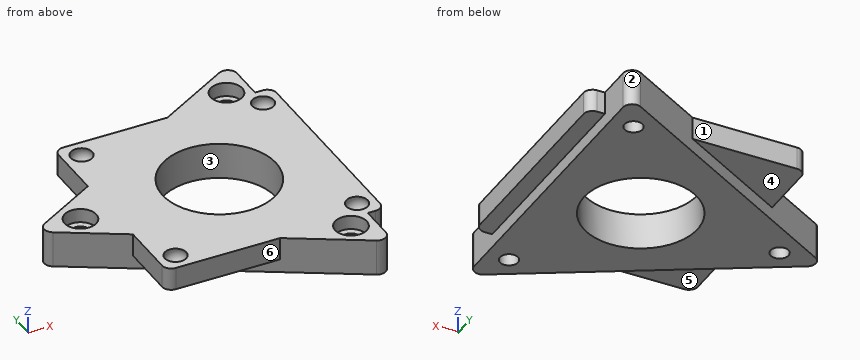
Autodesk Inventor part; units mm, degrees
ref_plane "YZ Plane" through (0, 0, 0) normal (1, 0, 0) x (0, 1, 0)
ref_plane "XZ Plane" through (0, 0, 0) normal (0, 1, 0) x (-1, 0, 0)
ref_plane "XY Plane" through (0, 0, 0) normal (0, 0, 1) x (1, 0, 0)
sketch "Sketch1" plane through (0, 0, 0) normal (0, 0, 1) x (1, 0, 0)
  line L0 (15.2998, 26.5) -> (15.2998, -26.5) construction
  line L1 (15.2998, -26.5) -> (-30.5996, 0) construction
  line L2 (-30.5996, 0) -> (15.2998, 26.5) construction
  line L3 (0, 48.0119) -> (0, -48.0119)
  circle A0 centre (0, 0) radius 12.5
  line L4 (24.9, -24.45) -> (-24.9, -24.45) construction
  line L5 (-24.9, -24.45) -> (-24.9, 24.45) construction
  line L6 (-24.9, 24.45) -> (24.9, 24.45) construction
  line L7 (24.9, 24.45) -> (24.9, -24.45) construction
  line L8 (24.9, -24.45) -> (-24.9, 24.45) construction
  line L9 (-24.9, -24.45) -> (24.9, 24.45) construction
  line L10 (20, -20) -> (-20, -20) construction
  line L11 (-20, -20) -> (-20, 20) construction
  line L12 (-20, 20) -> (20, 20) construction
  line L13 (20, 20) -> (20, -20) construction
  line L14 (20, -20) -> (-20, 20) construction
  line L15 (-20, -20) -> (20, 20) construction
  line L16 (-37.5996, -1.7321) -> (17.2998, -33.4282)
  line L17 (20.2998, -31.6962) -> (20.2998, 31.6962)
  line L18 (17.2998, 33.4282) -> (-37.5996, 1.7321)
  arc A1 (-37.5996, 1.7321) -> (-37.5996, -1.7321) centre (-36.5996, 0) ccw
  arc A2 (20.2998, 31.6962) -> (17.2998, 33.4282) centre (18.2998, 31.6962) ccw
  arc A3 (17.2998, -33.4282) -> (20.2998, -31.6962) centre (18.2998, -31.6962) ccw
  circle A4 centre (15.2998, 26.5) radius 2
  circle A5 centre (-30.5996, 0) radius 2
  circle A6 centre (15.2998, -26.5) radius 2
  dimension "d1" = 53
  dimension "d2" = 25
  dimension "d3" = 49.8
  dimension "d4" = 48.9
  dimension "d5" = 40
  dimension "d6" = 40
  dimension "d7" = 5
  dimension "d8" = 2
  dimension "d9" = 4
  dimension "d10" = 4
  dimension "d11" = 4
extrude "Extrusion1" add sketch "Sketch1" along normal blind 3 contours L18 A2 L17 A3 L16 L3 A0 | L3 A0 L16 A1 L18
sketch "Sketch3" plane through (0, 0, 3) normal (0, 0, 1) x (1, 0, 0)
  circle A0 centre (0, 0) radius 12.5
  circle A1 centre (15.2998, -26.5) radius 2
  circle A2 centre (-30.5996, 0) radius 2
  circle A3 centre (15.2998, 26.5) radius 2
  line L0 (-37.5996, -1.7321) -> (17.2998, -33.4282)
  arc A4 (17.2998, -33.4282) -> (20.2998, -31.6962) centre (18.2998, -31.6962) ccw
  line L1 (20.2998, -31.6962) -> (20.2998, 31.6962)
  arc A5 (20.2998, 31.6962) -> (17.2998, 33.4282) centre (18.2998, 31.6962) ccw
  line L2 (17.2998, 33.4282) -> (-37.5996, 1.7321)
  arc A6 (-37.5996, 1.7321) -> (-37.5996, -1.7321) centre (-36.5996, 0) ccw
  line L3 (22, -24) -> (-22, -24)
  line L4 (-24, -22) -> (-24, 22)
  line L5 (-22, 24) -> (22, 24)
  line L6 (24, 22) -> (24, -22)
  line L7 (24, -24) -> (-24, 24) construction
  line L8 (-24, -24) -> (24, 24) construction
  arc A7 (-22, 24) -> (-24, 22) centre (-22, 22) ccw
  arc A8 (-24, -22) -> (-22, -24) centre (-22, -22) ccw
  arc A9 (22, -24) -> (24, -22) centre (22, -22) ccw
  arc A10 (24, 22) -> (22, 24) centre (22, 22) ccw
  line L9 (17.2998, 33.4282) -> (-37.5996, 1.7321)
  line L10 (-37.5996, -1.7321) -> (17.2998, -33.4282)
  line L11 (20.2998, -31.6962) -> (20.2998, 31.6962)
  point P0 (20.2998, 24)
  point P1 (-24, 9.5838)
  point P2 (-24, -9.5838)
  point P3 (0.9697, -24)
  point P4 (20.2998, -24)
  dimension "d14" = 48
  dimension "d15" = 48
  dimension "d16" = 2
extrude "Extrusion2" add sketch "Sketch3" along normal blind 5 contours A0 | A1 | A3 | A6 L2 L4 L0 | L4 L2 L5 L1 L3 L0 | L0 L3 A8 L4 | L3 L1 A4 L0 | L4 A7 L5 L2 | L1 L5 A10 L6 A9 L3 | L2 A5 L1 L5
sketch "Sketch4" plane through (0, 0, 8) normal (0, 0, 1) x (1, 0, 0)
  circle A0 centre (0, 0) radius 12.5
  line L0 (20, -20) -> (-20, -20) construction
  line L1 (-20, -20) -> (-20, 20) construction
  line L2 (-20, 20) -> (20, 20) construction
  line L3 (20, 20) -> (20, -20) construction
  line L4 (20, -20) -> (-20, 20) construction
  line L5 (-20, -20) -> (20, 20) construction
  circle A1 centre (15.2998, 26.5) radius 2
  circle A2 centre (15.2998, -26.5) radius 2
  dimension "d19" = 40
  dimension "d20" = 40
extrude "Extrusion3" cut sketch "Sketch4" against normal through all
ref_plane "Work Plane1" through (-22, 0, 3) normal (0, 1, 0) x (1, 0, 0)
ref_plane "Work Plane2" through (0, -22, 3) normal (-1, 0, 0) x (0, 0, 1)
ref_plane "Work Plane3" through (-22, -20, 3) normal (0, 1, 0) x (1, 0, 0)
sketch "Sketch5" plane through (-22, -20, 3) normal (0, 1, 0) x (1, 0, 0)
  line L0 (22.9697, 0) -> (22.9697, -5)
  line L1 (22.9697, 0) -> (0, 0)
  line L2 (0, 0) -> (0, -5)
  line L3 (22.9697, -5) -> (0, -5)
  circle A0 centre (2, -4.2) radius 2.5
  line L4 (22, -11.7547) -> (22, 5.4591)
  line L5 (-0.5, -4.2) -> (4.5, -4.2)
  line L6 (0, 0) -> (0, -5)
  point P0 (22, 3)
  dimension "d24" = 5
  dimension "d25" = 20
  dimension "d26" = 0.8
revolve "Revolution1" cut sketch "Sketch5" angle 360 about axis through (-22.5, -20, 7.2) along (1, 0, 0) contours A0 L5 L2 L3 | L3 L2 L5 A0
pattern_linear "Rectangular Pattern1" count 2 spacing 40 along (1, 0, 0) count 2 spacing 40 along (0, 1, 0) of "Revolution1"
sketch "Sketch6" plane through (0, 0, 8) normal (0, 0, 1) x (1, 0, 0)
  circle A0 centre (20, 20) radius 2.3685
  circle A1 centre (-20, 20) radius 2.3685
  circle A2 centre (20, -20) radius 2.3685
  circle A3 centre (-20, -20) radius 2.3685
  circle A4 centre (15.2998, -26.5) radius 2
  circle A5 centre (15.2998, 26.5) radius 2
  circle A6 centre (0, 0) radius 12.5
  circle A7 centre (-30.5996, 0) radius 2
  line L0 (0.9697, 24) -> (-22, 24)
  arc A8 (-22, 24) -> (-24, 22) centre (-22, 22) ccw
  line L1 (-24, 22) -> (-24, 9.5838)
  line L2 (-24, 9.5838) -> (-37.5996, 1.7321)
  arc A9 (-37.5996, 1.7321) -> (-37.5996, -1.7321) centre (-36.5996, 0) ccw
  line L3 (-37.5996, -1.7321) -> (-24, -9.5838)
  line L4 (-24, -9.5838) -> (-24, -22)
  arc A10 (-24, -22) -> (-22, -24) centre (-22, -22) ccw
  line L5 (-22, -24) -> (0.9697, -24)
  line L6 (0.9697, -24) -> (17.2998, -33.4282)
  arc A11 (17.2998, -33.4282) -> (20.2998, -31.6962) centre (18.2998, -31.6962) ccw
  line L7 (20.2998, -31.6962) -> (20.2998, -24)
  line L8 (20.2998, -24) -> (22, -24)
  arc A12 (22, -24) -> (24, -22) centre (22, -22) ccw
  line L9 (24, -22) -> (24, 22)
  arc A13 (24, 22) -> (22, 24) centre (22, 22) ccw
  line L10 (22, 24) -> (20.2998, 24)
  line L11 (20.2998, 24) -> (20.2998, 31.6962)
  arc A14 (20.2998, 31.6962) -> (17.2998, 33.4282) centre (18.2998, 31.6962) ccw
  line L12 (17.2998, 33.4282) -> (0.9697, 24)
hole "Hole1" at (15.2998, 26.5, 8) at (15.2998, -26.5, 8) at (-30.5996, 0, 8) direction (0, 0, -1) diameter 2.8 depth 30 tip angle 118 counterbore diameter 7 counterbore depth 3.1
properties part number "20_Cube_Insert_Openflexure_Deltastage_Adapter"
Source: CAD feature listing. Evaluate the final solid. Frame: model axes, mm. Face numbers are marked on the shaded views. A direction names the side the tool comes from. Coordinates: 2 decimals unless noted, no trailing zeros. Loops run counter-clockwise (first coordinate to the right, second up) from the corner with the lowest first, then second, coordinate; pieces in that order, holes last. Notation, with made-up numbers: M 15,6 L 64,6 A22 cw 64,24 Z; hole C -20,74 d11. An arc over 180 degrees is marked long. Put each result on its own line as item: value. Start each with the question number.
1) Reachability of the marked faces 4, 5 and 6 from +Z, -Z, +X, -X, +Y, -Y: full face, straight path, thin tool, end or side. Return the list, or none.
2) Cut plane D-D on y = 26.5. Return the cut outline in (x, z), then the cut area to 3 significant figures.
3) Cut plane B-B on x = 0. Return the cut outline in (y, z).
4) Ray query, L1, parallel to Y at x = -0.5, z = 3.75; L2, parallel to X at y = -21.5, z = 5.5; L3, parallel to Y at x = 18.5, z = 6. Return the intervals inside material, ascending. Write a range as from..to.
5) Cut plane A-A on y = 0. Return the cut outline in (x, z).
6) Contact query for flat-ended pins moving along their axis: pin 1 Ø2 at (x, z) = (-28, 7) entering from +Y; pin 2 Ø4 at (y, z) = (-14.5, 4.5) entering from -X; pin 3 Ø5.5 at (x, y) = (15.3, 26.5) entering from +Z. Output: stop coordinate, or through.
7) Cut plane C-C on z = 1.75. Return the cut outline in (x, y), then the cut area to 3 significant figures.
8) Pull-direction query (X, two-part tool) for the marked faces 1, 2 and 3; classes: pulls with the +X half, pulls with the -X half, needs draft (parallel to the pull), parting line crosses it, or undercut.
The answers:
1. face 4: -Z, -X, +Y
1. face 5: -Z, -X, -Y
1. face 6: +Z, -Z, -X, -Y
2. outline: M 5.3,0 L 13.3,0 L 13.3,4.9 L 11.8,4.9 L 11.8,8 L 5.3,8 Z; M 17.3,0 L 20.3,0 L 20.3,8 L 18.8,8 L 18.8,4.9 L 17.3,4.9 Z
2. area: 78.7 mm²
3. outline: M -24,3 L -23.44,3 L -23.44,0 L -12.5,0 L -12.5,8 L -24,8 Z; M 12.5,0 L 23.44,0 L 23.44,3 L 24,3 L 24,8 L 12.5,8 Z
4. L1: y = -24..-12.49, 12.49..24
4. L2: x = -24..-21.05, -18.95..18.95, 21.05..24
4. L3: y = -33.69..-27.92, -25.08..-21.6, -18.4..18.4, 21.6..25.08, 27.92..33.69
5. outline: M -38.6,0 L -32.6,0 L -32.6,4.9 L -34.1,4.9 L -34.1,8 L -38.6,8 Z; M -28.6,0 L -12.5,0 L -12.5,8 L -27.1,8 L -27.1,4.9 L -28.6,4.9 Z; M 12.5,0 L 20.3,0 L 20.3,3 L 24,3 L 24,8 L 12.5,8 Z
6. pin 1: stops at y = 7.85
6. pin 2: stops at x = -24
6. pin 3: stops at z = 4.9
7. outline: M -37.6,-1.73 L 17.3,-33.43 A2 ccw 20.3,-31.7 L 20.3,31.7 A2 ccw 17.3,33.43 L -37.6,1.73 A2 ccw Z; hole C -30.6,0 d4; hole C 0,0 d25; hole C 15.3,-26.5 d4; hole C 15.3,26.5 d4
7. area: 1,600 mm²
8. face 1: needs draft
8. face 2: parting line crosses it
8. face 3: undercut
